Check sheet for the drawn part. Datum: minimum x, y, z corner. Units: mm. Coordinates: 2 decimals unless noted, no trailing zeros. Write each loop counter-clockwise with the first axis right and the second up, starting at its lowest first coordinate (ties: lowest second). Pieces come first, ordered by that corner, then holes. Notation, with made-up numbers: (83, 5) -> (134, 5) arc R38 cw to (134, 43) -> close; hole circle Ø8 at (83.5, 5.5). An arc over 180 degrees is marked (long way). Answer in a Markdown table with one row per item. Add a question column.
Q1. Thickness scan on line 1 (Y direction, x = 200, z = 1.65); line 2 (Y direction, x = 90, z = 3.35); line 3 (X direction, y = 139.5, z = 1.3). Record the ranges inside material, lowest first.
Q2. Section check A-A, the plane x = 255. Record the boundary of the cut face in (y, z), and give its area (3 significant figures).
Q3. Section check B-B, the plane y = 126. Record the boundary of the cut face in (x, z), and give its area (3 significant figures).
Q4. Section check C-C, the plane x = 35. Record the boundary of the cut face in (y, z), and give its area (3 significant figures).
Q5. Gauge pin test, flat ends, axial feed: P1, Ø9, axis at x = 310, y = 30, coming from the -Z side; P2, Ø1, axis at x = 274.5, z = 1.5, coming from the -Y side. Record the tip position at first contact, or that the pin passes through.
Q6. Section check D-D, the plane y = 174. Record the boundary of the cut face in (x, z).
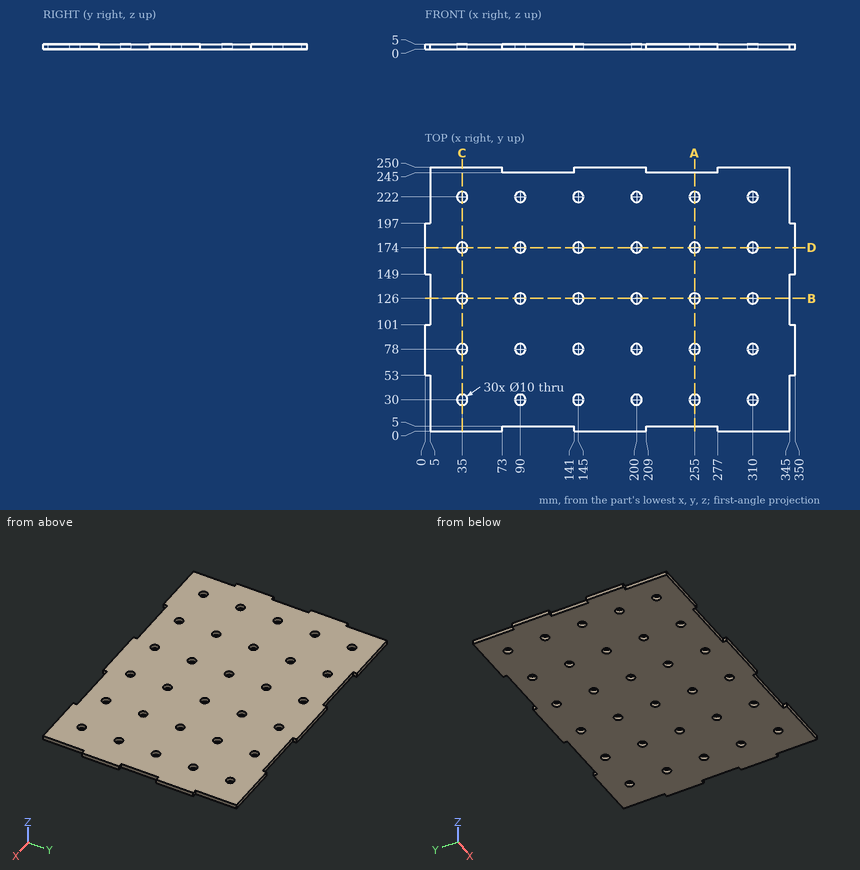
Calculated:
| question | item | result |
|---|---|---|
| 1 | line 1 | y = 0 to 25, 35 to 73, 83 to 121, 131 to 169, 179 to 217, 227 to 250 |
| 1 | line 2 | y = 5 to 25, 35 to 73, 83 to 121, 131 to 169, 179 to 217, 227 to 245 |
| 1 | line 3 | x = 5 to 345 |
| 2 | outline | (5, 0) -> (25, 0) -> (25, 5) -> (5, 5) -> close; (35, 0) -> (73, 0) -> (73, 5) -> (35, 5) -> close; (83, 0) -> (121, 0) -> (121, 5) -> (83, 5) -> close; (131, 0) -> (169, 0) -> (169, 5) -> (131, 5) -> close; (179, 0) -> (217, 0) -> (217, 5) -> (179, 5) -> close; (227, 0) -> (245, 0) -> (245, 5) -> (227, 5) -> close |
| 2 | area | 950 mm² |
| 3 | outline | (5, 0) -> (30, 0) -> (30, 5) -> (5, 5) -> close; (40, 0) -> (85, 0) -> (85, 5) -> (40, 5) -> close; (95, 0) -> (140, 0) -> (140, 5) -> (95, 5) -> close; (150, 0) -> (195, 0) -> (195, 5) -> (150, 5) -> close; (205, 0) -> (250, 0) -> (250, 5) -> (205, 5) -> close; (260, 0) -> (305, 0) -> (305, 5) -> (260, 5) -> close; (315, 0) -> (345, 0) -> (345, 5) -> (315, 5) -> close |
| 3 | area | 1,400 mm² |
| 4 | outline | (0, 0) -> (25, 0) -> (25, 5) -> (0, 5) -> close; (35, 0) -> (73, 0) -> (73, 5) -> (35, 5) -> close; (83, 0) -> (121, 0) -> (121, 5) -> (83, 5) -> close; (131, 0) -> (169, 0) -> (169, 5) -> (131, 5) -> close; (179, 0) -> (217, 0) -> (217, 5) -> (179, 5) -> close; (227, 0) -> (250, 0) -> (250, 5) -> (227, 5) -> close |
| 4 | area | 1,000 mm² |
| 5 | P1 | passes through |
| 5 | P2 | stops at y = 5 |
| 6 | outline | (0, 0) -> (30, 0) -> (30, 5) -> (0, 5) -> close; (40, 0) -> (85, 0) -> (85, 5) -> (40, 5) -> close; (95, 0) -> (140, 0) -> (140, 5) -> (95, 5) -> close; (150, 0) -> (195, 0) -> (195, 5) -> (150, 5) -> close; (205, 0) -> (250, 0) -> (250, 5) -> (205, 5) -> close; (260, 0) -> (305, 0) -> (305, 5) -> (260, 5) -> close; (315, 0) -> (350, 0) -> (350, 5) -> (315, 5) -> close |
